The model under review builds one solid part; all positions refer to its coordinate system, in mm. Face numbers are marked on the shaded views. Round coordinates to 2 decimals unless told otherwise and drop trailing zeros. Loops run counter-clockwise (first coordinate to the right, second up) from the corner with the lowest first, then second, coordinate; pieces in that order, holes last. Notation, with made-up numbers: (53, 26) -> (107, 26) arc R29 ccw to (107, 65) -> close; hole circle Ø5 at (71.5, 44.5). An arc over 180 degrees is marked (long way). Return JSON: item names as keys, results as strings. Group by question number.
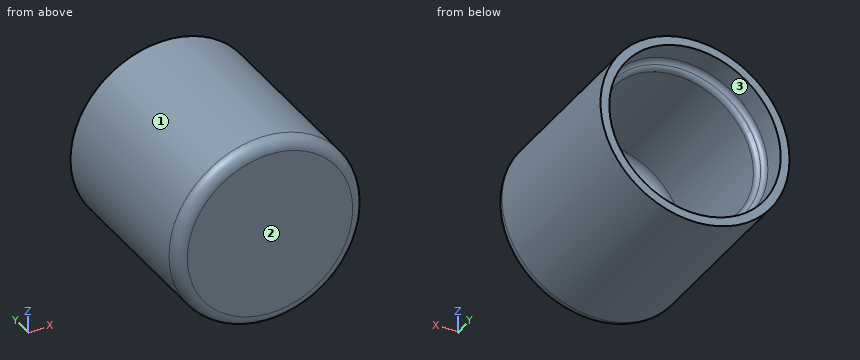
Autodesk Inventor part; units mm, degrees
ref_plane "YZ Plane" through (0, 0, 0) normal (1, 0, 0) x (0, 1, 0)
ref_plane "XZ Plane" through (0, 0, 0) normal (0, 1, 0) x (-1, 0, 0)
ref_plane "XY Plane" through (0, 0, 0) normal (0, 0, 1) x (1, 0, 0)
sketch "Sketch1" plane through (0, 0, 0) normal (0, 1, 0) x (-1, 0, 0)
  circle A0 centre (0, 0) radius 12.7
  dimension "d1" = 25.4
extrude "Extrusion1" add sketch "Sketch1" against normal blind 25.4
shell "Shell1" thickness 2.286 removed faces 1 at (-0.1664, 0, 2.8072)
sketch "Sketch2" plane through (0, 0, 0) normal (0, 1, 0) x (1, 0, 0)
  circle A0 centre (0, 0) radius 11.5189
  dimension "d5" = 23.0378
extrude "Extrusion2" cut sketch "Sketch2" against normal blind 3.81
fillet "Fillet1" radius 1.5875 1 edges at (12.7, -25.4, 0)
fillet "Fillet2" radius 1.5875 1 edges at (10.414, -23.114, 0)
fillet "Fillet3" radius 0.7937 1 edges at (10.414, -3.81, 0)
fillet "Fillet4" radius 0.7937 1 edges at (-11.5189, -3.81, 0)
properties part number "Bolt Cap"
1. For P1, Ø14, axis at x = -4, z = 1, coming from the +Y side; P2, Ø1, axis at x = 1, y = -16.5, coming from the +Z side; P3, Ø2, axis at x = 3, y = -9.5, coming from the +Z side, all flat-tipped, find the tip position at first contact; note any pin that passes through.
2. Wall thickness on line 1 (Z direction, x = 0, y = -2.4); line 2 (Z direction, x = 0, y = -12.75); line 3 (X direction, y = -12.75, z = 2): over which ranges is each line inside the solid? List them lowest first.
3. We need section A-A, the plane y = -19.75. Write out the cut boundary in (x, z), then the cut area to 3 significant figures.
4. Draft analysis for pull direction Z (two halves, no side actions). For the marked faces 1, 2 and 3, state which applies: pulls with the +Z half, pulls with the -Z half, needs draft (parallel to the pull), parting line crosses it, or undercut.
Check sheet entries:
{
 "1": {"P1": "stops at y = -3.78", "P2": "stops at z = 12.69", "P3": "stops at z = 12.54"},
 "2": {"line 1": "z = -12.7 to -11.52, 11.52 to 12.7", "line 2": "z = -12.7 to -10.41, 10.41 to 12.7", "line 3": "x = -12.54 to -10.22, 10.22 to 12.54"},
 "3": {"outline": "circle Ø25.4 at (0, 0); hole circle Ø20.83 at (0, 0)", "area": "166 mm²"},
 "4": {"face 1": "parting line crosses it", "face 2": "needs draft", "face 3": "undercut"}
}
